Here's how the part is built. I have some questions about the finished solid (model axes, mm). Face numbers are marked on the shaded views. A direction names the side the tool comes from. Give positions to 0.01 mm unless a question says otherwise; leave off trailing zeros. Loops run counter-clockwise (first coordinate to the right, second up) from the corner with the lowest first, then second, coordinate; pieces in that order, holes last. Notation, with made-up numbers: (51, -25) - (99, -25) arc R21 ccw to (99, 3) - close; hole circle Ø9 at (42, 14). An arc over 180 degrees is marked (long way). Use one line per item in the form item = value.
from build123d import *

# Parameters (mm, degrees)
SKETCH1_W           = 5.162383308
SKETCH1_H           = 20.435052184
BOSS_EXTRUDE1_DEPTH = 1.27
SKETCH2_W           = 0.838933851
SKETCH2_H           = 3.882140463
CUT_EXTRUDE1_DEPTH  = 3.81
SKETCH3_W           = 0.823014711
SKETCH3_H           = 2.56348928
BOSS_EXTRUDE2_DEPTH = 2.54


with BuildPart() as part:
    # Sketch1 → Boss-Extrude1 (new body)
    with BuildSketch(Plane.XY):
        with Locations((-34.98361032, 7.835499756)):
            Rectangle(SKETCH1_W, SKETCH1_H)
    extrude(amount=BOSS_EXTRUDE1_DEPTH)

    # Sketch2 → Cut-Extrude1 (cut)
    with BuildSketch(Plane.ZY.offset(37.564801974)):
        with Locations((0.611191145, 14.932897959)):
            Rectangle(SKETCH2_W, SKETCH2_H)
    extrude(amount=-CUT_EXTRUDE1_DEPTH, mode=Mode.SUBTRACT)

    # Sketch3 → Boss-Extrude2 (add)
    with BuildSketch(Plane(origin=(-32.402418666, 0, 0), x_dir=(0, 0, -1), z_dir=(1, 0, 0))):
        with Locations((-0.670761293, -1.100281696)):
            Rectangle(SKETCH3_W, SKETCH3_H)
    extrude(amount=BOSS_EXTRUDE2_DEPTH)


solid = part.part
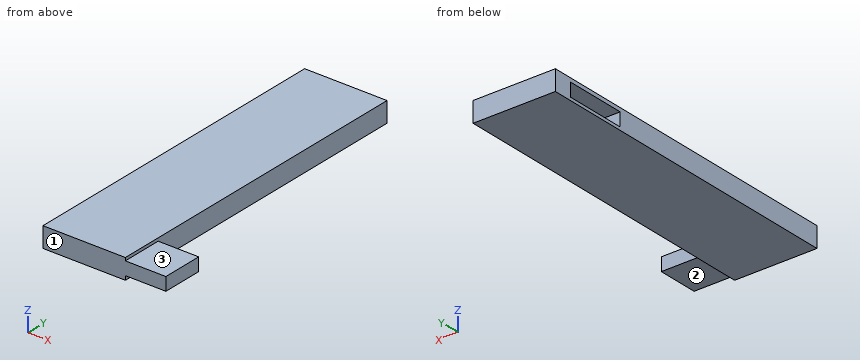
(1) For P1, Ø0.8, axis at x = -31, y = -1, coming from the +Z side; P2, Ø0.7, axis at x = -31.5, z = 0.5, coming from the +Y side, each with a flat end and sliding along its axis, tell me the tip position at first contact or that it passes through.
Geometry says:
P1 = 1.08
P2 = 0.18
(2) If I drill on probe 1 along Y at (x, z) = (-34.75, 0.75); probe 2 along Z at (x, y) = (-36.5, 14.5); probe 3 along X at (y, z) = (14.25, 0.25), over which ranges is the centre line in solid material (lowest first)?
Geometry says:
probe_1 = -2.38 to 12.99, 16.87 to 18.05
probe_2 = 0 to 0.19, 1.03 to 1.27
probe_3 = -33.75 to -32.4
(3) If we section it at B-B (x = -35.5): List the corners of the cut face in (y, z) for me, plus the area to 3 significant figures.
Geometry says:
outline = (-2.38, 0) - (18.05, 0) - (18.05, 1.27) - (-2.38, 1.27) - close; hole (12.99, 0.19) - (16.87, 0.19) - (16.87, 1.03) - (12.99, 1.03) - close
area = 22.7 mm²
(4) If we section it at A-A (y = -0.5): List the corners of the cut face in (x, z) for me.
Geometry says:
outline = (-37.56, 0) - (-32.4, 0) - (-32.4, 0.26) - (-29.86, 0.26) - (-29.86, 1.08) - (-32.4, 1.08) - (-32.4, 1.27) - (-37.56, 1.27) - close
(5) For the marked faces 1, 2 and 3, which set-ups out of +Z, -Z, +X, -X, +Y, -Y let a thin tool reach every point of the face, with its end or its side?
Geometry says:
face_1 = +Z, -Z, +X, -X, -Y
face_2 = -Z, +X, +Y, -Y
face_3 = +Z, +X, +Y, -Y
(6) If we section it at D-D (y = 14.5): List the corners of the cut face in (x, z) for me.
Geometry says:
outline = (-37.56, 0) - (-32.4, 0) - (-32.4, 1.27) - (-37.56, 1.27) - (-37.56, 1.03) - (-33.75, 1.03) - (-33.75, 0.19) - (-37.56, 0.19) - close
(7) If we section it at C-C (x = -32): List the corners of the cut face in (y, z) for me, plus the area to 3 significant figures.
Geometry says:
outline = (-2.38, 0.26) - (0.18, 0.26) - (0.18, 1.08) - (-2.38, 1.08) - close
area = 2.11 mm²
